Geometry: final body of the model. Coordinates: model frame, mm. A direction names the side the tool comes from. Give positions to 0.01 mm unless a question says otherwise; leave off trailing zeros. Write each loop counter-clockwise with the first axis right and the second up, starting at its lowest first coordinate (ties: lowest second). Pieces come first, ordered by that corner, then holes.
Autodesk Inventor part; units mm, degrees
ref_plane "YZ Plane" through (0, 0, 0) normal (1, 0, 0) x (0, 1, 0)
ref_plane "XZ Plane" through (0, 0, 0) normal (0, 1, 0) x (-1, 0, 0)
ref_plane "XY Plane" through (0, 0, 0) normal (0, 0, 1) x (1, 0, 0)
sketch "Sketch1" plane through (0, 0, 0) normal (0, 0, 1) x (1, 0, 0)
  line L0 (63.5, -6.35) -> (63.5, 6.35)
  line L1 (63.5, 6.35) -> (-63.5, 6.35)
  line L2 (-63.5, 6.35) -> (-63.5, -6.35)
  line L3 (0, 0) -> (0, -40) construction
  line L4 (-63.5, -6.35) -> (-21.6259, -6.35)
  line L5 (21.6259, -6.35) -> (63.5, -6.35)
  line L6 (-63.5, -6.35) -> (-6.9307, -0.6931) construction
  line L7 (0, 0) -> (63.5, 6.35) construction
  line L8 (63.5, -6.35) -> (6.9307, -0.6931) construction
  line L9 (0, 0) -> (-63.5, 6.35) construction
  arc A0 (-21.6259, -6.35) -> (21.6259, -6.35) centre (0, -40) ccw
  line L10 (63.5, 0) -> (-63.5, 0) construction
  dimension "d0" = 127
  dimension "d1" = 12.7
  dimension "d2" = 40
  dimension "d31" = 6.35
  dimension "d32" = 40
extrude "Extrusion1" add sketch "Sketch1" against normal blind 25.4
sketch "Sketch2" plane through (0, 0, 0) normal (0, 0, 1) x (1, 0, 0)
  arc A0 (-21.6259, -6.35) -> (21.6259, -6.35) centre (0, -40) ccw
  circle A1 centre (0, -40) radius 35
  point P0 (0, 0)
  dimension "d6" = 70
extrude "Extrusion2" cut sketch "Sketch2" against normal blind 2.794
sketch "Sketch3" plane through (0, -40, -2.794) normal (0, 0, 1) x (1, 0, 0)
  circle A0 centre (0, 0) radius 35
  circle A1 centre (0, 0) radius 31
  circle A2 centre (0, 0) radius 24
  point P0 (0, 40)
  dimension "d9" = 62
  dimension "d10" = 48
extrude "Extrusion3" cut sketch "Sketch3" against normal blind 2 contours A0 | A1
sketch "Sketch4" plane through (0, -40, -4.794) normal (0, 0, 1) x (1, 0, 0)
  circle A0 centre (0, 0) radius 35 construction
  line L0 (0, 0) -> (34.925, 0) construction
  circle A1 centre (29.5, 0) radius 5
  point P0 (0, 40)
  dimension "d33" = 29.5
  dimension "d34" = 10
extrude "Extrusion4" cut sketch "Sketch4" against normal through all
sketch "Sketch5" plane through (-63.5, -6.35, 0) normal (0, -1, 0) x (1, 0, 0)
  line L0 (0, 0) -> (0, -25.4) construction
  line L1 (0, -12.7) -> (127, -12.7) construction
  line L2 (127, 0) -> (127, -25.4) construction
  point P0 (63.5, 0)
  point P1 (12.7, -12.7)
  point P2 (114.3, -12.7)
  dimension "d15" = 12.7
  dimension "d16" = 12.7
hole "Hole1" at (-50.8, -6.35, -12.7) at (50.8, -6.35, -12.7) direction (0, 1, 0) diameter 6.7564 end through all counterbore diameter 8.0264 counterbore depth 9.525
sketch "Sketch6" plane through (0, 0, -25.4) normal (0, 0, -1) x (-1, 0, 0)
  circle A0 centre (-29.5, -40) radius 5
  line L0 (63.5, -6.35) -> (63.5, 6.35)
  line L1 (63.5, 6.35) -> (-63.5, 6.35)
  line L2 (-63.5, 6.35) -> (-63.5, -6.35)
  line L3 (-63.5, -6.35) -> (-21.6259, -6.35)
  arc A1 (-21.6259, -6.35) -> (21.6259, -6.35) centre (0, -40) ccw
  line L4 (21.6259, -6.35) -> (63.5, -6.35)
  line L5 (1.1662, -29.21) -> (1.1662, -40.2844)
  line L6 (3.1474, -29.21) -> (1.1662, -29.21)
  line L7 (3.1474, -40.2844) -> (3.1474, -29.21)
  line L8 (3.1474, -40.2844) -> (16.4443, -40.2844)
  line L9 (16.4443, -40.2844) -> (16.4443, 3.9878)
  arc A2 (16.4443, 3.9878) -> (14.0821, 6.35) centre (14.0821, 3.9878) ccw
  line L10 (-9.7685, 6.35) -> (14.0821, 6.35)
  arc A3 (-9.7685, 6.35) -> (-12.1307, 3.9878) centre (-9.7685, 3.9878) ccw
  line L11 (-12.1307, -40.2844) -> (-12.1307, 3.9878)
  line L12 (-12.1307, -40.2844) -> (1.1662, -40.2844)
  line L13 (13.4998, -8.7122) -> (13.4998, -24.5872)
  line L14 (13.4998, -24.5872) -> (-9.1862, -24.5872)
  line L15 (-9.1862, -24.5872) -> (-9.1862, -8.7122)
  line L16 (-9.1862, -8.7122) -> (13.4998, -8.7122)
  circle A4 centre (-8.9557, 0.8128) radius 1.6256
  circle A5 centre (13.2693, -34.1122) radius 1.6256
  circle A6 centre (13.2693, 0.8128) radius 1.6256
  circle A7 centre (-8.9557, -34.1122) radius 1.6256
  point P0 (0, 0)
hole "Hole2" at (-13.2693, 0.8128, -25.4) at (-13.2693, -34.1122, -25.4) at (8.9557, -34.1122, -25.4) at (8.9557, 0.8128, -25.4) direction (0, 0, 1) diameter 3.5052 depth 12.7 tip angle 118 counterbore diameter 4.8514 counterbore depth 7.1374
sketch "Sketch8" plane through (0, -40, -2.794) normal (0, 0, 1) x (1, 0, 0)
  circle A0 centre (-16.2398, -9.376) radius 1.905
  circle A1 centre (0, 18.7521) radius 1.905
  circle A2 centre (16.2398, -9.3761) radius 1.905
  line L0 (22.8154, -16.5062) -> (18.8007, -20.9651)
  line L1 (18.8007, -20.9651) -> (15.8281, -18.2886)
  line L2 (15.8281, -18.2886) -> (19.8429, -13.8297)
  line L3 (19.8429, -13.8297) -> (22.8154, -16.5062)
  line L4 (27.533, 5.9104) -> (28.1602, -0.0568)
  line L5 (28.1602, -0.0568) -> (24.1821, -0.4749)
  line L6 (24.1821, -0.4749) -> (23.5549, 5.4922)
  line L7 (23.5549, 5.4922) -> (27.533, 5.9104)
  line L8 (14.0309, 24.4158) -> (18.885, 20.8891)
  line L9 (18.885, 20.8891) -> (16.5339, 17.6531)
  line L10 (16.5339, 17.6531) -> (11.6798, 21.1798)
  line L11 (11.6798, 21.1798) -> (14.0309, 24.4158)
  line L12 (-8.756, 26.7644) -> (-2.8871, 28.0119)
  line L13 (-2.8871, 28.0119) -> (-2.0554, 24.0993)
  line L14 (-2.0554, 24.0993) -> (-7.9243, 22.8518)
  line L15 (-7.9243, 22.8518) -> (-8.756, 26.7644)
  line L16 (-25.7487, 11.4019) -> (-22.7487, 16.5981)
  line L17 (-22.7487, 16.5981) -> (-19.2846, 14.5981)
  line L18 (-19.2846, 14.5981) -> (-22.2846, 9.4019)
  line L19 (-22.2846, 9.4019) -> (-25.7487, 11.4019)
  line L20 (-25.7025, -11.5056) -> (-27.5566, -5.7993)
  line L21 (-27.5566, -5.7993) -> (-23.7524, -4.5632)
  line L22 (-23.7524, -4.5632) -> (-21.8983, -10.2696)
  line L23 (-21.8983, -10.2696) -> (-25.7025, -11.5056)
  line L24 (-8.648, -26.7995) -> (-14.1293, -24.3591)
  line L25 (-14.1293, -24.3591) -> (-12.5023, -20.7049)
  line L26 (-12.5023, -20.7049) -> (-7.021, -23.1453)
  line L27 (-7.021, -23.1453) -> (-8.648, -26.7995)
  line L28 (3, -24) -> (3, -28)
  line L29 (3, -28) -> (-3, -28)
  line L30 (-3, -28) -> (-3, -24)
  line L31 (-3, -24) -> (3, -24)
  line L32 (-18.8007, -20.9651) -> (-22.8154, -16.5062)
  line L33 (-22.8154, -16.5062) -> (-19.8429, -13.8297)
  line L34 (-19.8429, -13.8297) -> (-15.8281, -18.2886)
  line L35 (-15.8281, -18.2886) -> (-18.8007, -20.9651)
  line L36 (-28.1602, -0.0568) -> (-27.533, 5.9104)
  line L37 (-27.533, 5.9104) -> (-23.5549, 5.4922)
  line L38 (-23.5549, 5.4922) -> (-24.1821, -0.4749)
  line L39 (-24.1821, -0.4749) -> (-28.1602, -0.0568)
  line L40 (-18.885, 20.8891) -> (-14.0309, 24.4158)
  line L41 (-14.0309, 24.4158) -> (-11.6798, 21.1798)
  line L42 (-11.6798, 21.1798) -> (-16.5339, 17.6531)
  line L43 (-16.5339, 17.6531) -> (-18.885, 20.8891)
  line L44 (2.8871, 28.0119) -> (8.756, 26.7644)
  line L45 (8.756, 26.7644) -> (7.9243, 22.8518)
  line L46 (7.9243, 22.8518) -> (2.0554, 24.0993)
  line L47 (2.0554, 24.0993) -> (2.8871, 28.0119)
  line L48 (22.7487, 16.5981) -> (25.7487, 11.4019)
  line L49 (25.7487, 11.4019) -> (22.2846, 9.4019)
  line L50 (22.2846, 9.4019) -> (19.2846, 14.5981)
  line L51 (19.2846, 14.5981) -> (22.7487, 16.5981)
  line L52 (27.5566, -5.7993) -> (25.7025, -11.5056)
  line L53 (25.7025, -11.5056) -> (21.8983, -10.2696)
  line L54 (21.8983, -10.2696) -> (23.7524, -4.5632)
  line L55 (23.7524, -4.5632) -> (27.5566, -5.7993)
  line L56 (14.1293, -24.3591) -> (8.648, -26.7995)
  line L57 (8.648, -26.7995) -> (7.021, -23.1453)
  line L58 (7.021, -23.1453) -> (12.5023, -20.7049)
  line L59 (12.5023, -20.7049) -> (14.1293, -24.3591)
  line L60 (5, 5) -> (5, -5)
  line L61 (5, -5) -> (-5, -5)
  line L62 (-5, -5) -> (-5, 5)
  line L63 (-5, 5) -> (5, 5)
  circle A3 centre (0, 0) radius 34
  point P0 (0, 40)
hole "Hole3" at (0, -21.2479, -2.794) at (-16.2398, -49.376, -2.794) at (16.2398, -49.3761, -2.794) direction (0, 0, -1) diameter 3.5052 depth 12.7 tip angle 118 counterbore diameter 4.8514 counterbore depth 7.1374
sketch "Sketch10" plane through (0, -40, -2.794) normal (0, 0, 1) x (1, 0, 0)
  line L0 (-4, -4) -> (-4, 4)
  line L1 (-4, 4) -> (4, 4)
  line L2 (4, 4) -> (4, -4)
  line L3 (4, -4) -> (-4, -4)
  circle A0 centre (10.5, -12.5) radius 1.1
  circle A1 centre (10.5, 0.08) radius 1.1
  circle A2 centre (-10.5, 0.08) radius 1.1
  circle A3 centre (-10.5, -12.5) radius 1.1
  arc A4 (-12.5, -12.5) -> (-10.5, -14.5) centre (-10.5, -12.5) ccw
  line L4 (-10.5, -14.5) -> (10.5, -14.5)
  arc A5 (10.5, -14.5) -> (12.5, -12.5) centre (10.5, -12.5) ccw
  line L5 (12.5, -12.5) -> (12.5, 7.542)
  arc A6 (12.5, 7.542) -> (10.5, 9.542) centre (10.5, 7.542) ccw
  line L6 (10.5, 9.542) -> (-10.5, 9.542)
  arc A7 (-10.5, 9.542) -> (-12.5, 7.542) centre (-10.5, 7.542) ccw
  line L7 (-12.5, 7.542) -> (-12.5, -12.5)
  line L8 (-13.5, 10.542) -> (13.5, 10.542)
  circle A8 centre (0, 0) radius 24
  line L9 (-13.5, -15.5) -> (-13.5, 10.542)
  line L10 (-13.5, -15.5) -> (13.5, -15.5)
  line L11 (13.5, 10.542) -> (13.5, -15.5)
  point P0 (0, 40)
  dimension "d54" = 1
  dimension "d55" = 1
  dimension "d56" = 1
  dimension "d57" = 1
ref_plane "Work Plane1" through (0, -40, -9.794) normal (0, 0, 1) x (1, 0, 0)
sketch "Sketch11" plane through (0, -40, -9.794) normal (0, 0, 1) x (1, 0, 0)
  line L0 (-4, -4) -> (-4, 4)
  line L1 (-4, 4) -> (4, 4)
  line L2 (4, 4) -> (4, -4)
  line L3 (4, -4) -> (-4, -4)
  circle A0 centre (10.5, -12.5) radius 1.1
  circle A1 centre (10.5, 0.08) radius 1.1
  circle A2 centre (-10.5, 0.08) radius 1.1
  circle A3 centre (-10.5, -12.5) radius 1.1
  arc A4 (-12.5, -12.5) -> (-10.5, -14.5) centre (-10.5, -12.5) ccw
  line L4 (-10.5, -14.5) -> (10.5, -14.5)
  arc A5 (10.5, -14.5) -> (12.5, -12.5) centre (10.5, -12.5) ccw
  line L5 (12.5, -12.5) -> (12.5, 7.542)
  arc A6 (12.5, 7.542) -> (10.5, 9.542) centre (10.5, 7.542) ccw
  line L6 (10.5, 9.542) -> (-10.5, 9.542)
  arc A7 (-10.5, 9.542) -> (-12.5, 7.542) centre (-10.5, 7.542) ccw
  line L7 (-12.5, 7.542) -> (-12.5, -12.5)
  point P0 (0, 40)
hole "Hole4" at (-10.5, -39.92, -9.794) at (10.5, -39.92, -9.794) at (10.5, -52.5, -9.794) at (-10.5, -52.5, -9.794) direction (0, 0, -1) diameter 3.5052 depth 12.7 tip angle 118 counterbore diameter 4.8514 counterbore depth 7.1374
extrude "Extrusion7" cut sketch "Sketch10" against normal blind 7 contours L0 L1 L2 L3 | A0 | A1 | A2 | A3 | L7 A7 L6 A6 L5 A5 L4 A4 | L8 L11 L10 L9
properties part number "basicMount"
Q1. Section C-C on x = -6. Output: boundary loops of the cut face in (y, z).
Filled sheet:
outline: (-79.55, -25.4) - (6.35, -25.4) - (6.35, 0) - (-5.52, 0) - (-5.52, -4.79) - (-16.76, -4.79) - (-16.76, -2.79) - (-29.46, -2.79) - (-29.46, -9.79) - (-55.5, -9.79) - (-55.5, -2.79) - (-63.24, -2.79) - (-63.24, -4.79) - (-74.48, -4.79) - (-74.48, 0) - (-79.55, 0) - close
Q2. Section A-A on x = 50.8. Output: boundary loops of the cut face in (y, z) (3 decimals), plus the area to 3 significant figures.
Filled sheet:
outline: (-6.35, -25.4) - (6.35, -25.4) - (6.35, -16.078) - (3.175, -16.078) - (3.175, -16.713) - (-6.35, -16.713) - close; (-6.35, -8.687) - (3.175, -8.687) - (3.175, -9.322) - (6.35, -9.322) - (6.35, 0) - (-6.35, 0) - close
area: 225 mm2
Q3. Pin query (flat end, axial travel): P1, Ø21, axis at x = 3.5, y = -40, coming from the +Z side; P2, Ø4.5, axis at x = 8.96, y = 0.81, coming from the +Z side; P3, Ø4, axis at x = 0, y = -21.25, coming from the +Z side; P4, Ø12, axis at y = -29.5, z = -3.5, coming from the -X side. Return the tip coordinate at first contact, or that it passes through.
Filled sheet:
P1: stops at z = -2.79
P2: stops at z = 0
P3: stops at z = -9.93
P4: stops at x = -39.75
Q4. Section B-B on x = -27.5. Output: boundary loops of the cut face in (y, z), plus the area to 3 significant figures.
Filled sheet:
outline: (-69.05, -25.4) - (-10.95, -25.4) - (-10.95, 0) - (-18.35, 0) - (-18.35, -4.79) - (-61.65, -4.79) - (-61.65, 0) - (-69.05, 0) - close; (-6.35, -25.4) - (6.35, -25.4) - (6.35, 0) - (-6.35, 0) - close
area: 1,590 mm2
Q5. Pull-direction query (Y, two-part tool) for faces 4 (the flat face through (-0.3, -4.6, 0)), 5 (the flat face through (10, -42, -16.931)), 6 (the flat face through (-13.5, -43, -6)); classes: released by +Y, released by -Y, zero draft, split by the parting line, or undercut.
Filled sheet:
face 4: zero draft
face 5: undercut
face 6: undercut
Q6. Access query for faces 1 (the flat face through (7, -35, -18.263)), 2 (the cylindrical face through (16.9, -51, -12.8)), 3 (the cylindrical face through (54.1, 4.78, -11.97)). Directions: +Z, -Z, +X, -X, +Y, -Y. A direction counts if a zero-diameter tool reaches every point of the face in a straight line with its end or side. Return the directions, or none.
Filled sheet:
face 1: -Z
face 2: +Z
face 3: +Y, -Y
Q7. Ray query, line 1 along X through (y, z) = (-39.92, -12.25); line 2 along X through (y, z) = (-39.92, -18.8); line 3 along Y through (x, z) = (27, -18.25). Return the intervals inside material, ascending.
Filled sheet:
line 1: x = -40 to -12.93, -8.07 to 8.07, 12.93 to 24.5, 34.5 to 40
line 2: x = -40 to -12.25, -8.75 to 8.75, 12.25 to 24.5, 34.5 to 40
line 3: y = -69.51 to -44.33, -35.67 to -10.49, -6.35 to 6.35
